Verification items for the finished model (mm, model axes). Face numbers are marked on the shaded views. A direction names the side the tool comes from. Give positions to 0.01 mm unless a question says otherwise; leave off trailing zeros. Write each loop counter-clockwise with the first axis right and the second up, starting at its lowest first coordinate (ties: lowest second). Pieces come first, ordered by that corner, then holes. Notation, with made-up numbers: (-35.75, -17) -> (16.25, -17) arc R17 ccw to (16.25, 8) -> close; hole circle Ø3 at (13, 80). An arc over 180 degrees is marked (long way). Answer as CSV lines item,"result".
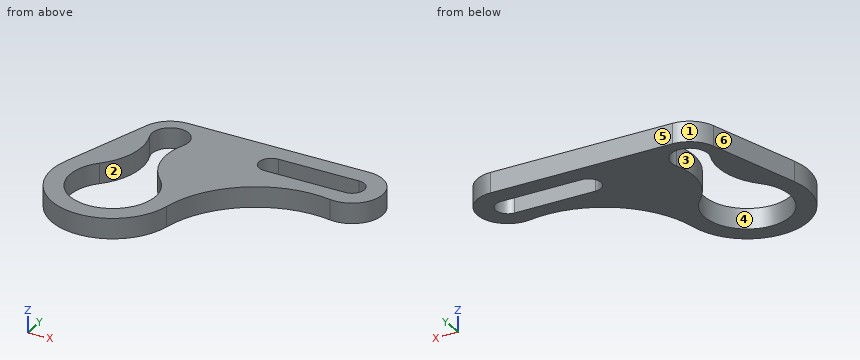
```python
from build123d import *

# Parameters (mm, degrees)
BOSS_EXTRUDE1_DEPTH = 5


with BuildPart() as part:
    # Sketch1 → Boss-Extrude1 (new, symmetric)
    with BuildSketch(Plane.XY):
        with BuildLine():
            Line((0, 65), (90, 65))
            ThreePointArc((90, 65), (104.943418217, 48.698365648), (87.406551135, 35.225900265))
            ThreePointArc((87.406551135, 35.225900265), (50.100874494, 26.949083525), (29.535645594, -5.25791207))
            ThreePointArc((29.535645594, -5.25791207), (-7.143700144, -29.137047693), (-28.618176043, 9))
            Line((-28.618176043, 9), (-14.309088021, 54.5))
            ThreePointArc((-14.309088021, 54.5), (-8.874119675, 62.093386622), (0, 65))
        make_face()
        with BuildLine():
            Line((50, 56), (90, 56))
            ThreePointArc((90, 56), (96, 50), (90, 44))
            Line((90, 44), (50, 44))
            ThreePointArc((50, 44), (44, 50), (50, 56))
        make_face(mode=Mode.SUBTRACT)
        with BuildLine():
            ThreePointArc((8.382229724, 46.723076923), (0, 59), (-8.382229724, 46.723076923))
            ThreePointArc((-8.382229724, 46.723076923), (-6.937432482, 29.759413292), (-14.956527547, 14.741176471))
            ThreePointArc((-14.956527547, 14.741176471), (0, -21), (14.956527547, 14.741176471))
            ThreePointArc((14.956527547, 14.741176471), (6.937432482, 29.759413292), (8.382229724, 46.723076923))
        make_face(mode=Mode.SUBTRACT)
    extrude(amount=BOSS_EXTRUDE1_DEPTH, both=True)


solid = part.part
```
1) Tool access check on the marked faces 1 and 2. Record the directions out of +Z, -Z, +X, -X, +Y, -Y that give a thin tool (end or side, any length) a straight path to the whole face; none if there is none.
Reported:
face 1,"+Z, -Z, -X, +Y"
face 2,"+Z, -Z"
2) Section check D-D (y = 50). Record the boundary of the cut face in (x, z).
Reported:
outline,"(-15.72, -5) -> (-9, -5) -> (-9, 5) -> (-15.72, 5) -> close; (9, -5) -> (44, -5) -> (44, 5) -> (9, 5) -> close; (96, -5) -> (105, -5) -> (105, 5) -> (96, 5) -> close"
3) Section check B-B (x = 57). Record the boundary of the cut face in (y, z), and give its area (3 significant figures).
Reported:
outline,"(30.99, -5) -> (44, -5) -> (44, 5) -> (30.99, 5) -> close; (56, -5) -> (65, -5) -> (65, 5) -> (56, 5) -> close"
area,"220 mm²"
4) Depth check by flat-ended pin: pin 1 (5 mm diameter, centred on y = 37, z = 0, fed in from +X); pin 2 (6 mm diameter, centred on x = 11.5, z = -2.5, fed in from -Y); pin 3 (4 mm diameter, centred on x = 77.5, z = 1.5, fed in from -Y). Enter the tip coordinate at first touch or a pass-through.
Reported:
pin 1,"x = 100.71"
pin 2,"y = -28.77"
pin 3,"y = 35.87"
5) Section check A-A (y = 0). Record the boundary of the cut face in (x, z).
Reported:
outline,"(-30, -5) -> (-21, -5) -> (-21, 5) -> (-30, 5) -> close; (21, -5) -> (30.77, -5) -> (30.77, 5) -> (21, 5) -> close"
6) Section check C-C (z = -1). Record the boundary of the cut face in (x, y).
Reported:
outline,"(-28.62, 9) arc R30 ccw (long way) to (29.54, -5.26) arc R50 cw to (87.41, 35.23) arc R15 ccw (long way) to (90, 65) -> (0, 65) arc R15 ccw to (-14.31, 54.5) -> close; hole (-14.96, 14.74) arc R21 ccw (long way) to (14.96, 14.74) arc R30 cw to (8.38, 46.72) arc R9 ccw (long way) to (-8.38, 46.72) arc R30 cw to start; hole (50, 44) -> (90, 44) arc R6 ccw to (90, 56) -> (50, 56) arc R6 ccw to start"
7) Draft check along X on the marked faces 3, 4, 5 and 6. Enter one of: +X half, -X half, draft (parallel to the pull), parting line (faces both ways), or undercut.
Reported:
face 3,"undercut"
face 4,"undercut"
face 5,"draft"
face 6,"-X half"
8) Scan lines: line 1 along X through (y, z) = (-12, 0.5); line 2 along Y through (x, z) = (74, 4); line 3 along Y through (x, z) = (63, -1.75). Record each from-to range of solid material in increasing order.
Reported:
line 1,"-27.5 to -17.23, 17.23 to 27.5"
line 2,"35.75 to 44, 56 to 65"
line 3,"33.43 to 44, 56 to 65"
